Autodesk Inventor part; units mm, degrees
ref_plane "Work Plane1" through (0, -4.064, 8.255) normal (0, 0, -1) x (0, 1, 0)
ref_plane "Work Plane2" through (0, 0, 4.1275) normal (0, 0, -1) x (-1, 0, 0)
ref_plane "YZ Plane" through (0, 0, 0) normal (1, 0, 0) x (0, 1, 0)
sketch "Sketch2" plane through (0, 0, 0) normal (0, 0, 1) x (1, 0, 0)
  arc A0 (4.191, -4.318) -> (4.191, 4.318) centre (4.191, 0) ccw
  arc A1 (4.191, 4.318) -> (4.191, -4.318) centre (4.191, 0) ccw
  circle A2 centre (4.191, 0) radius 1.397
  line L0 (8.509, 0) -> (8.509, 4.318)
  line L1 (8.509, 4.318) -> (4.191, 4.318)
  line L2 (8.509, 0) -> (8.509, -4.318)
  line L3 (8.509, -4.318) -> (4.191, -4.318)
  point P0 (0, 0)
ref_plane "Work Plane1" through (0, -4.064, 8.255) normal (0, 0, -1) x (0, 1, 0)
extrude "Extrusion1" add sketch "Sketch2" along normal up to surface (8.255 mm away)
ref_plane "Work Plane2" through (0, 0, 4.1275) normal (0, 0, -1) x (-1, 0, 0)
sketch "Sketch3" plane through (4.191, -4.318, 0) normal (0, -1, 0) x (1, 0, 0)
  circle A0 centre (20.32, 4.1275) radius 12.7
  line L0 (40.4876, 4.1275) -> (-11.7856, 4.1275)
  line L1 (4.318, 0) -> (4.318, 8.255)
  circle A1 centre (20.32, 4.1275) radius 11.176
  line L2 (0, 14.2875) -> (4.064, 14.2875)
  line L3 (4.064, -6.0325) -> (0, -6.0325)
  line L4 (0, 0) -> (4.318, 0)
  line L5 (4.318, 0) -> (4.318, -6.0386)
  line L6 (4.318, 8.255) -> (4.318, 14.2875)
  arc A2 (4.318, 14.2875) -> (16.3873, 16.2033) centre (4.318, 53.2638) ccw
  arc A3 (16.3963, -7.9512) -> (4.318, -6.0386) centre (4.318, -45.1333) ccw
  point P0 (-4.191, 0)
  dimension "d2" = 25.4
  dimension "d3" = 0
  dimension "d4" = 16.002
  dimension "d5" = 1.524
  dimension "d8" = 0
  dimension "d9" = 0.0061
extrude "Extrusion2" add sketch "Sketch3" against normal up to surface (8.636 mm away) contours L0 A1 A0 | A0 L0 A1 | A0 L0 L1 L6 A2 | A3 L5 L1 L0 A0
fillet "Fillet1" radius 0.254 12 edges at (8.509, 4.318, -3.0193) (8.509, 4.318, 11.2712) (8.509, 0, -6.0386) (8.509, -4.318, -3.0193) (8.509, -4.318, 11.2712) (8.509, 0, 14.2875) (37.211, -4.318, 4.1322) (14.6234, -4.318, -6.5197) (14.6192, -4.318, 14.7694) (37.211, 4.318, 4.1322) (14.6234, 4.318, -6.5197) (14.6192, 4.318, 14.7694)
properties part number "wrenchB"
CAD build for the part. Positions are in the model's coordinates, mm. A direction names the side the tool comes from. Round coordinates to 2 decimals unless told otherwise and drop trailing zeros. Order: outer loops, then holes, each group sorted by start corner. A loop starts at its lowest first (then second) coordinate and runs counter-clockwise, first axis right, second up.
Q1. Slice it at B-B (x = 3.5). Write the cut outline in (y, z) (3 decimals), and give its area (3 significant figures).
Q2. Which spindle directions (+Z, -Z, +X, -X, +Y, -Y) get a long thin tool onto all of the face, cutting with end or side? Do faces 1 (the flat face through (13, 4.318, 3)), 2 (the flat face through (8.509, 0, -3)), 3 (the flat face through (8.509, 0, 11)). Say none if no direction does.
Q3. Slice it at A-A (y = 0). State how many separate pieces and enclosed holes the cut face has, and give its area (3 significant figures).
Q4. Wall check: L1, parallel to X at y = -0.5, z = 2.5; L2, parallel to Z at x = 4.5, y = -3 (3 decimals); L3, parallel to Z at x = 21, y = 0.5. Give the ranges that are in metal, low to high.
Q5. Drop flat-ended pins along their axis: pin 1 (2 mm diameter, centred on x = 30, y = 2, fed in from +Z); pin 2 (1.7 mm diameter, centred on y = -1, z = -2, fed in from -X); pin 3 (1.5 mm diameter, centred on x = 19.5, y = 0.5, fed in from -Z). Give the stop position or say it passes through.
Q6. Two-plate mould, pull along X, no slides. Class faces 4 (the cylindrical face through (37.207, -0.057, 3.797)), 5 (the flat face through (6, 0, 8.255)), 6 (the cylindrical face through (5.48, 0.54, 4.07)): pulls with the +X half, pulls with the -X half, needs draft (parallel to the pull), parting line crosses it, or undercut.
Results below:
1. outline: (-4.262, 0) - (-1.214, 0) - (-1.214, 8.255) - (-4.262, 8.255) - close; (1.214, 0) - (4.262, 0) - (4.262, 8.255) - (1.214, 8.255) - close
1. area: 50.3 mm2
2. face 1: +Z, -Z, +X, -X, +Y
2. face 2: -Z, -X, +Y, -Y
2. face 3: +Z, -X, +Y, -Y
3. separate pieces: 2
3. enclosed holes: 1
3. area: 268 mm2
4. L1: x = -0.1 to 2.89, 5.5 to 13.45, 35.57 to 37.11
4. L2: z = 0 to 8.255
4. L3: z = -8.08 to -6.48, 14.74 to 16.33
5. pin 1: stops at z = 16.01
5. pin 2: stops at x = 8.51
5. pin 3: stops at z = -7.84
6. face 4: parting line crosses it
6. face 5: needs draft
6. face 6: undercut
